Read the model definition and answer for the solid it produces. Units are mm, in the model's axes. Coordinates: 2 decimals unless noted, no trailing zeros. Order: outer loops, then holes, each group sorted by start corner. A loop starts at its lowest first (then second) coordinate and runs counter-clockwise, first axis right, second up. Notation, with made-up numbers: M -30.75,69.25 L 9.25,69.25 A18 ccw 9.25,89.25 Z; hole C 22.5,4 d4. An arc over 180 degrees is marked long. One line per question, with ' | ' between items. Start each with the question number.
1) Consider probe 1 along X at (y, z) = (4.75, 0); probe 2 along Z at (x, y) = (-23.5, 5.7); probe 3 along X at (y, z) = (2.15, 3). Determine where each line is inside the solid, lowest interval first.
2) Find section B-B, the plane z = -0.75. Write down the section's boundary in (x, y).
3) Find section D-D, the plane x = 25. Write down the section's boundary in (y, z).
4) Given P1, Ø6, axis at x = 0, z = 0, coming from the -Y side; P2, Ø2, axis at x = -67.5, y = 2.5, coming from the -Z side; P3, Ø1.8, axis at x = -66, y = 4, coming from the +Z side, each flat-ended and moving along its own axis, determine where each tip first touches the part or whether it passes through.
5) Find section A-A, the plane x = 0. Write down the section's boundary in (y, z).
6) Find section C-C, the plane y = 4.35. Write down the section's boundary in (x, z).
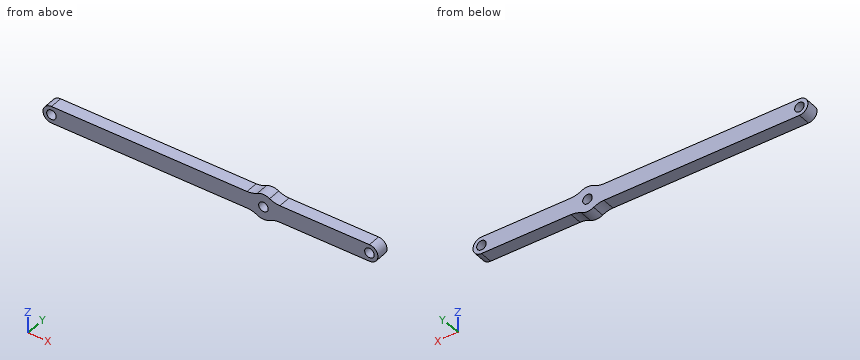
from build123d import *

# Parameters (mm, degrees)
SKETCH1_R           = 2.25
BOSS_EXTRUDE1_DEPTH = 6
FILLET1_R           = 10


with BuildPart() as part:
    # Sketch1 → Boss-Extrude1 (new body)
    with BuildSketch(Plane(origin=(0, 0, 0), x_dir=(1, 0, 0), z_dir=(0, 1, 0))):
        with BuildLine():
            Line((-100, 4), (-4.472135955, 4))
            ThreePointArc((-4.472135955, 4), (0, 6), (4.472135955, 4))
            Line((4.472135955, 4), (50, 4))
            ThreePointArc((50, 4), (54, 0), (50, -4))
            Line((50, -4), (4.472135955, -4))
            ThreePointArc((4.472135955, -4), (0, -6), (-4.472135955, -4))
            Line((-4.472135955, -4), (-100, -4))
            ThreePointArc((-100, -4), (-104, 0), (-100, 4))
        make_face()
        with Locations(Location((0, 0, 0), (0, 0, 270))):
            Circle(SKETCH1_R, mode=Mode.SUBTRACT)
        with Locations(Location((50, 0, 0), (0, 0, 270))):
            Circle(SKETCH1_R, mode=Mode.SUBTRACT)
        with Locations(Location((-100, 0, 0), (0, 0, 270))):
            Circle(SKETCH1_R, mode=Mode.SUBTRACT)
    extrude(amount=BOSS_EXTRUDE1_DEPTH)

    # Fillet1
    fillet1_edges = [part.edges().sort_by_distance(p)[0] for p in [
        (4.472135955, 3, -4),
        (4.472135955, 3, 4),
        (-4.472135955, 3, 4),
        (-4.472135955, 3, -4),
    ]]
    fillet(fillet1_edges, radius=FILLET1_R)


solid = part.part
Report:
1) probe 1: x = -104 to -102.25, -97.75 to -2.25, 2.25 to 47.75, 52.25 to 54 | probe 2: z = -4 to 4 | probe 3: x = -102.65 to 52.65
2) outline: M -103.93,0 L -102.12,0 L -102.12,6 L -103.93,6 Z; M -97.88,0 L -2.12,0 L -2.12,6 L -97.88,6 Z; M 2.12,0 L 47.88,0 L 47.88,6 L 2.12,6 Z; M 52.12,0 L 53.93,0 L 53.93,6 L 52.12,6 Z
3) outline: M 0,-4 L 6,-4 L 6,4 L 0,4 Z
4) P1: stops at y = 0 | P2: stops at z = -4 | P3: stops at z = 4
5) outline: M 0,-6 L 6,-6 L 6,-2.25 L 0,-2.25 Z; M 0,2.25 L 6,2.25 L 6,6 L 0,6 Z
6) outline: M -100,-4 L -7.75,-4 A10 cw -2.9,-5.25 A6 ccw 2.9,-5.25 A10 cw 7.75,-4 L 50,-4 A4 ccw 50,4 L 7.75,4 A10 cw 2.9,5.25 A6 ccw -2.9,5.25 A10 cw -7.75,4 L -100,4 A4 ccw Z; hole C -100,0 d4.5; hole C 0,0 d4.5; hole C 50,0 d4.5
